Autodesk Inventor part; units mm, degrees
ref_plane "XZ Plane" through (0, 0, 0) normal (0, 1, 0) x (-1, 0, 0)
ref_plane "XY Plane" through (0, 0, 0) normal (0, 0, 1) x (1, 0, 0)
sketch "Sketch1" plane through (0, 0, 0) normal (0, 1, 0) x (-1, 0, 0)
  line L0 (0, 0) -> (0, -12.7)
  line L1 (0, -12.7) -> (-17.78, -12.7)
  line L2 (-17.78, -12.7) -> (-17.78, -9.525)
  line L3 (-17.78, -9.525) -> (-45.72, -9.525)
  line L4 (-45.72, -9.525) -> (-45.72, -12.7)
  line L5 (-45.72, -12.7) -> (-63.5, -12.7)
  line L6 (-63.5, -12.7) -> (-63.5, 0)
  line L7 (-63.5, 0) -> (-60.325, 0)
  line L8 (-60.325, 0) -> (-60.325, -6.35)
  line L9 (-60.325, -6.35) -> (-3.175, -6.35)
  line L10 (-3.175, -6.35) -> (-3.175, 0)
  line L11 (-3.175, 0) -> (0, 0)
  dimension "d0" = 12.7
  dimension "d1" = 3.175
  dimension "d2" = 17.78
  dimension "d3" = 63.5
  dimension "d4" = 3.175
  dimension "d5" = 3.175
revolve "Revolution1" add sketch "Sketch1" angle 180 about axis through (63.5, 0, 0) along (1, 0, 0)
fillet "Fillet1" radius 1.5875 6 edges at (63.5, 12.7, 0) (17.78, 9.525, 0) (17.78, 12.7, 0) (0, 12.7, 0) (45.72, 9.525, 0) (45.72, 12.7, 0)
sketch "Sketch2" plane through (0, 0, 0) normal (-1, 0, 0) x (0, 0, 1)
  circle A0 centre (0, 0) radius 1.397
  dimension "d8" = 2.794
extrude "Extrusion1" cut sketch "Sketch2" against normal through all
sketch "Sketch3" plane through (3.175, 0, 6.35) normal (0, -1, 0) x (1, 0, 0)
  line L0 (0, 0) -> (57.15, 0) construction
  line L1 (57.15, -12.7) -> (0, -12.7) construction
  line L2 (0, -4.953) -> (0, -7.747) construction
  line L3 (0, -6.35) -> (10.7724, -6.35) construction
  line L4 (10.7724, -6.35) -> (46.1567, -6.35) construction
  line L5 (46.1567, -6.35) -> (56.929, -6.35) construction
  line L6 (0, -12.7) -> (0, 0)
  line L7 (28.575, 0) -> (28.575, -12.7) construction
  line L8 (57.15, -7.747) -> (57.15, -4.953)
  line L9 (28.575, -10.7083) -> (28.575, -12.7)
  line L10 (57.15, -7.747) -> (28.575, -7.747) construction
  line L11 (28.575, -10.7083) -> (38.743, -10.7083)
  line L12 (40.775, -8.8314) -> (40.775, -12.7)
  line L13 (40.775, -12.7) -> (28.575, -12.7)
  line L14 (28.575, -12.7) -> (28.575, -10.7083)
  line L15 (38.743, -10.7083) -> (38.743, -12.7)
  line L16 (36.4298, -11.4703) -> (36.4298, -10.7083) construction
  line L17 (29.337, -10.5155) -> (28.575, -10.5155) construction
  line L18 (37.981, -10.5156) -> (38.743, -10.5156) construction
  line L19 (38.743, -10.7083) -> (38.743, -8.8314)
  line L20 (38.743, -8.8314) -> (40.775, -8.8314)
  circle A0 centre (54.9756, -10.5155) radius 1.55
  arc A1 (57.15, -7.747) -> (52.197, -12.7) centre (57.15, -12.7) ccw
  line L21 (57.15, -12.7) -> (53.6477, -9.1977) construction
  line L22 (57.15, -7.747) -> (57.15, -12.7)
  line L23 (57.15, -12.7) -> (52.197, -12.7)
  point P0 (-3.175, -6.35)
  dimension "d27" = 2.032
  dimension "d28" = 3.1
extrude "Extrusion3" add sketch "Sketch3" against normal up to next
mirror "Mirror1" about plane through (0, 0, 0) normal (0, 0, 1) of "Extrusion3"
ref_plane "Work Plane1" through (31.75, 0, -9.525) normal (1, 0, 0) x (0, 1, 0)
mirror "Mirror2" about plane through (31.75, 0, -9.525) normal (1, 0, 0) of "Extrusion3", "Mirror1"
sketch "Sketch4" plane through (19.3675, 0, -9.525) normal (0, -1, 0) x (1, 0, 0)
  line L0 (22.5505, 3.175) -> (2.2145, 3.175)
  line L1 (2.2145, 3.175) -> (2.2145, 15.8996)
  line L2 (2.2145, 15.8996) -> (22.5505, 15.8996)
  line L3 (22.5505, 15.8996) -> (22.5505, 3.175)
  point P0 (-19.3675, 9.525)
  point P1 (36.0045, 3.175)
  point P2 (40.9575, 3.175)
  point P3 (24.5825, 7.0436)
extrude "Extrusion4" cut sketch "Sketch4" against normal blind 1.6002
ref_plane "Work Plane2" through (31.75, 0, -9.525) normal (1, 0, 0) x (0, 1, 0)
properties part number "resistor"
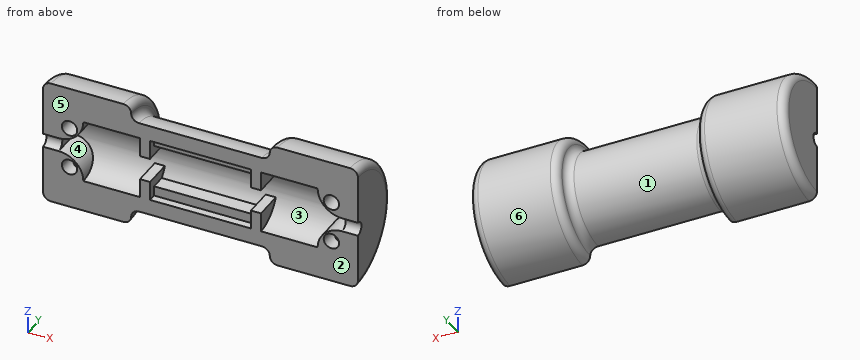
Design review of the part built by this model. Coordinates are the model's own, in mm. Face numbers are marked on the shaded views. A direction names the side the tool comes from. Round coordinates to 2 decimals unless told otherwise and drop trailing zeros. Write each loop counter-clockwise with the first axis right and the second up, starting at its lowest first coordinate (ties: lowest second). Pieces come first, ordered by that corner, then holes. Notation, with made-up numbers: M 23,51 L 55,51 A19 ccw 55,63 Z; hole C -7.5,17 d6. An arc over 180 degrees is marked long. One line per item, written item: value. Start each with the question number.
1. Take a section at A-A on x = 39. State the section outline as (y, z) points (3 decimals), then the cut area to 3 significant figures.
2. Draft analysis for pull direction Z (two halves, no side actions). For the marked faces 3, 4, 5 and 6, state which applies: pulls with the +Z half, pulls with the -Z half, needs draft (parallel to the pull), parting line crosses it, or undercut.
3. To check wall thickness, follow probe 1 along X at (y, z) = (5.25, -1.25) (3 decimals); probe 2 along X at (y, z) = (4.25, -10.25); probe 3 along Z at (x, y) = (16.5, 5). State the ranges of each line that lie inside material, in increasing order. Write a range as from..to.
4. Clearance check with flat-ended pins moving along their axes: P1, Ø1.5, axis at y = 8, z = -4, coming from the -X side; P2, Ø5, axis at x = 47, y = 9.5, coming from the -Z side; P3, Ø3, axis at x = 18.5, y = 5.5, coming from the +Z side; P4, Ø10, axis at x = 48.5, z = 8, coming from the +Y side. State where each tip first meets the part, or that it passes through.
5. For the marked faces 1 and 2, list the 3-axis set-ups (+Z, -Z, +X, -X, +Y, -Y) from which the entire face can be reached by the end or side of a thin tool; tool diameter is ignored.
Computed:
1. outline: M 0,-9.525 A9.525 ccw 0,9.525 L 0,6.375 L 1.6,6.375 L 1.6,4.358 L 4.618,4.358 A6.35 cw 4.618,-4.358 L 1.6,-4.358 L 1.6,-6.35 L 0,-6.35 Z
1. area: 85.5 mm²
2. face 3: undercut
2. face 4: undercut
2. face 5: needs draft
2. face 6: parting line crosses it
3. probe 1: x = 0..3.175, 60.325..63.5
3. probe 2: x = 0..17.78, 45.72..63.5
3. probe 3: z = -11.64..-3.91, 3.91..11.64
4. P1: stops at x = 0
4. P2: stops at z = -10.59
4. P3: stops at z = 11.39
4. P4: stops at y = 12.34
5. face 1: +Y
5. face 2: +Z, -Z, +X, -X, -Y
